from build123d import *

# Parameters (mm, degrees)
F0_R     = 13.732641
F1_DEPTH = 36.576
F0_W     = 102.870002
F0_H     = 76.46276
F2_DEPTH = 23.368


with BuildPart() as f1:
    # F0 (on Top) → F1 (new body)
    with BuildSketch(Plane.XY):
        with BuildLine():
            ThreePointArc((28.772071, 0), (2.561897, 26.694094), (-23.648277, 0))
            ThreePointArc((-23.648277, 0), (2.561897, -26.210174), (28.772071, 0))
        make_face()
        with Locations((2.561897, 0.479534)):
            Circle(F0_R, mode=Mode.SUBTRACT)
    extrude(amount=F1_DEPTH)

    # F0 (on Top) → F2 (join)
    with BuildSketch(Plane.XY):
        Rectangle(F0_W, F0_H)
        with BuildLine():
            ThreePointArc((28.772071, 0), (2.561897, -26.210174), (-23.648277, 0))
            ThreePointArc((-23.648277, 0), (2.561897, 26.694094), (28.772071, 0))
        make_face(mode=Mode.SUBTRACT)
    extrude(amount=F2_DEPTH)


solid = f1.part
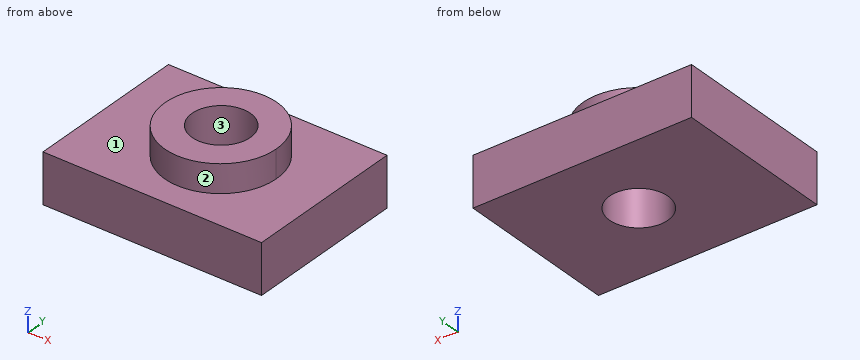
Could you check a few things on this model? Use its own coordinates, in mm. Face numbers are marked on the shaded views. Give positions to 0.01 mm unless a question says otherwise; leave off trailing zeros. Write each loop counter-clockwise with the first axis right and the second up, starting at its lowest first coordinate (ties: lowest second). Pieces come first, ordered by that corner, then holes. Notation, with made-up numbers: (-16.75, 76) -> (-2.75, 76) arc R17 ccw to (-2.75, 93) -> close; hole circle Ø10 at (-31, 7). An arc over 180 degrees is marked (long way). Answer as a JSON object with one key per item and string values.
Q1. Please list where these lines run through material, in increasing order: L1, parallel to Z at x = 28.5, y = -29.5; L2, parallel to Y at x = -10, z = 16; L3, parallel to X at y = 13, z = 4 (3 decimals).
Taken from the geometry:
{"L1": "z = 0 to 23.37", "L2": "y = -38.23 to -5.07, 6.03 to 38.23", "L3": "x = -51.435 to -3.079, 8.203 to 51.435"}
Q2. Suppose I cut it at A-A on x = -5.5. Write out the boundary of the cut face in (y, z).
Taken from the geometry:
{"outline": "(-38.23, 0) -> (-10.64, 0) -> (-10.64, 36.58) -> (-24.94, 36.58) -> (-24.94, 23.37) -> (-38.23, 23.37) -> close; (11.6, 0) -> (38.23, 0) -> (38.23, 23.37) -> (25.42, 23.37) -> (25.42, 36.58) -> (11.6, 36.58) -> close"}
Q3. Will these pins go through, and if not, where does the flat tip stop? pin 1 Ø10 at (y, z) = (-16.5, 30) entering from -X; pin 2 Ø5 at (y, z) = (-6, 32) entering from +X.
Taken from the geometry:
{"pin 1": "stops at x = -20.99", "pin 2": "stops at x = 28.54"}
Q4. We'd pull the mould along Y, two halves only. Please class the marked faces 1, 2 and 3: released by +Y, released by -Y, zero draft, split by the parting line, or undercut.
Taken from the geometry:
{"face 1": "zero draft", "face 2": "released by -Y", "face 3": "undercut"}
Q5. Suppose I cut it at B-B on z = 20. Write out the boundary of the cut face in (x, y) (3 decimals), then the cut area to 3 significant figures.
Taken from the geometry:
{"outline": "(-51.435, -38.231) -> (51.435, -38.231) -> (51.435, 38.231) -> (-51.435, 38.231) -> close; hole circle Ø27.465 at (2.562, 0.48)", "area": "7,270 mm²"}
Q6. Suppose I cut it at C-C on x = -28. Write out the boundary of the cut face in (y, z), then the cut area to 3 significant figures.
Taken from the geometry:
{"outline": "(-38.23, 0) -> (38.23, 0) -> (38.23, 23.37) -> (-38.23, 23.37) -> close", "area": "1,790 mm²"}
